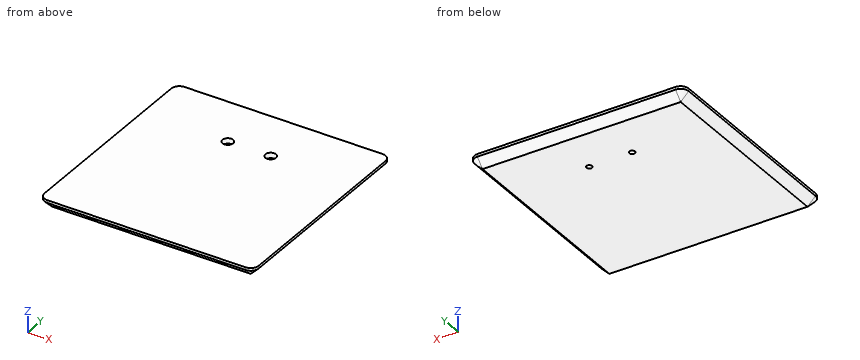
Autodesk Inventor part; units mm, degrees
ref_plane "YZ Plane" through (0, 0, 0) normal (1, 0, 0) x (0, 1, 0)
ref_plane "XZ Plane" through (0, 0, 0) normal (0, 1, 0) x (-1, 0, 0)
ref_plane "XY Plane" through (0, 0, 0) normal (0, 0, 1) x (1, 0, 0)
sketch "Sketch1" plane through (0, 0, 0) normal (0, 0, 1) x (1, 0, 0)
  circle A0 centre (5, 0) radius 1.1
  circle A1 centre (-11, 0) radius 1.1
  line L0 (-11, 0) -> (5, 0) construction
  line L1 (-43, 20) -> (37, 20)
  line L2 (-3, 22.8039) -> (-3, -25.7358) construction
  line L3 (37, 20) -> (37, -60)
  line L4 (37, -60) -> (-43, -60)
  line L5 (-43, -60) -> (-43, 20)
  point P0 (0, 0)
  point P1 (-3, 0)
  point P2 (-3, 20)
  dimension "d0" = 80
  dimension "d1" = 80
  dimension "d2" = 20
extrude "Extrusion1" add sketch "Sketch1" along normal blind 4 contours A0 | A1 | L1 L3 L4 L5
fillet "Fillet1" radius 3 4 edges at (-43, 20, 2) (-43, -60, 2) (37, -60, 2) (37, 20, 2)
sketch "Sketch2" plane through (0, 0, 4) normal (0, 0, 1) x (1, 0, 0)
  circle A0 centre (-11, 0) radius 1.1
  circle A1 centre (5, 0) radius 1.1
  point P0 (0, 0)
hole "Hole1" at (-11, 0, 4) at (5, 0, 4) direction (0, 0, -1) diameter 2.1 end through all counterbore diameter 4 counterbore depth 2
chamfer "Chamfer1" distance 3 angle 45 8 edges at (-43, -20, 0) (-42.1213, 19.1213, 0) (-3, 20, 0) (36.1213, 19.1213, 0) (37, -20, 0) (36.1213, -59.1213, 0) (-3, -60, 0) (-42.1213, -59.1213, 0)
equation "\"d1\" = d0"
properties part number "Touchplate"
Could you check a few things on this model? Use its own coordinates, in mm. Round coordinates to 2 decimals unless told otherwise and drop trailing zeros. Loops run counter-clockwise (first coordinate to the right, second up) from the corner with the lowest first, then second, coordinate; pieces in that order, holes last. Notation, with made-up numbers: (3.5, -30.75) - (13.5, -30.75) arc R17 ccw to (13.5, -11.75) - close; hole circle Ø1 at (67, 66). An arc over 180 degrees is marked (long way). Answer in a Markdown table with one row per item. Add a question column.
(1) If we section it at B-B (y = 0): Please give me the cut outline in (x, z).
(2) If we section it at A-A (x = -11): Please give me the cut outline in (y, z), plus the area to 3 significant figures.
(3) I need wall thicknesses on line 1 along X through (y, z) = (0, 3.3); line 2 along X through (y, z) = (0, 1.35); line 3 along Y through (x, z) = (5, 3.4). Which ranges of each line are inside material? Lowest first, please.
(4) I'm going to push flat-ended pins straight in: pin 1 (1.9 mm diameter, centred on x = -11, y = 0, fed in from +Z); pin 2 (1.5 mm diameter, centred on x = 23, z = 1, fed in from -Y). Where does each tip first touch, or does it pass through?
Model answer:
| question | item | result |
|---|---|---|
| 1 | outline | (-43, 3) - (-40, 0) - (-12.05, 0) - (-12.05, 2) - (-13, 2) - (-13, 4) - (-43, 4) - close; (-9.95, 0) - (3.95, 0) - (3.95, 2) - (3, 2) - (3, 4) - (-9, 4) - (-9, 2) - (-9.95, 2) - close; (6.05, 0) - (34, 0) - (37, 3) - (37, 4) - (7, 4) - (7, 2) - (6.05, 2) - close |
| 2 | outline | (-60, 3) - (-57, 0) - (-1.05, 0) - (-1.05, 2) - (-2, 2) - (-2, 4) - (-60, 4) - close; (1.05, 0) - (17, 0) - (20, 3) - (20, 4) - (2, 4) - (2, 2) - (1.05, 2) - close |
| 2 | area | 299 mm² |
| 3 | line 1 | x = -43 to -13, -9 to 3, 7 to 37 |
| 3 | line 2 | x = -41.35 to -12.05, -9.95 to 3.95, 6.05 to 35.35 |
| 3 | line 3 | y = -60 to -2, 2 to 20 |
| 4 | pin 1 | passes through |
| 4 | pin 2 | stops at y = -58.75 |
